Here's how the part is built. I have some questions about the finished solid (model axes, mm). Face numbers are marked on the shaded views. A direction names the side the tool comes from. Round coordinates to 2 decimals unless told otherwise and drop trailing zeros. Write each loop counter-clockwise with the first axis right and the second up, starting at its lowest first coordinate (ties: lowest second). Pieces come first, ordered by that corner, then holes. Notation, with made-up numbers: (-35.75, 44) -> (1.25, 44) arc R5 ccw to (1.25, 52) -> close; hole circle Ø6 at (69, 68). An arc over 180 degrees is marked (long way). Put each result on its own line as item: value. Start each with the question number.
1. Suppose I cut it at D-D (x = 22.5). Please give me the cut outline in (y, z).
2. For pin 1 (1.5 mm diameter, centred on x = -31.5, z = 7.5, fed in from +Y); pin 2 (3.5 mm diameter, centred on y = -1.5, z = 18.5, fed in from -X); pin 3 (2.5 mm diameter, centred on x = 22, y = 1.5, fed in from +Z), each with a flat end and sliding along its axis, tell me the tip position at first contact or that it passes through.
3. Suppose I cut it at C-C (y = -14). Please give me the cut outline in (x, z), then the cut area to 3 significant figures.
4. Suppose I cut it at B-B (z = 9). Count the separate pieces of the cut face and the enclosed holes in it, then the cut area to 3 significant figures.
5. I need wall thicknesses on probe 1 along X at (y, z) = (-18, 11); probe 2 along X at (y, z) = (-14.5, 11.5); probe 3 along X at (y, z) = (-11.75, 1). Which ranges of each line are inside material? Lowest first, please. Write a range as from..to.
6. Suppose I cut it at A-A (y = 0). Please give me the cut outline in (x, z), then the cut area to 3 significant figures.
7. Which directions (+Z, -Z, +X, -X, +Y, -Y) give clear straight access to the entire face, cutting with the end or side of a thin tool? Please do the marked faces 1, 2 and 3.
8. We'd pull the mould along Y, two halves only. Please class the marked faces 4, 5 and 6: +Y half, -Y half, draft (parallel to the pull), parting line (faces both ways), or undercut.
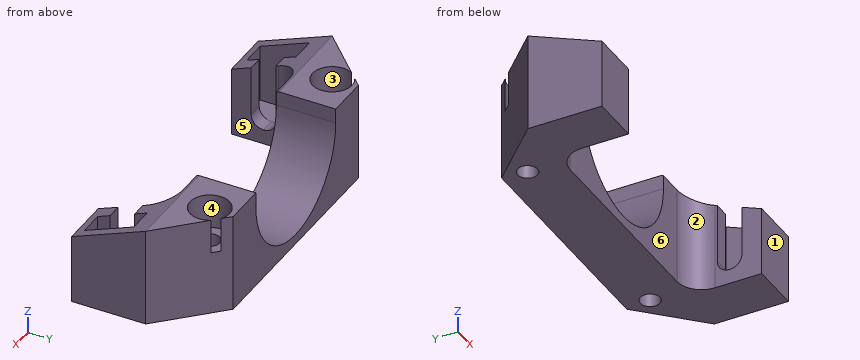
```python
from build123d import *

# Parameters (mm, degrees)
SKETCH1_R               = 2
BOSS_EXTRUDE1_DEPTH     = 20
SKETCH2_W               = 5.5
SKETCH2_H               = 5
SKETCH2_W_2             = 3
SKETCH2_W_3             = 2.5
CUT_EXTRUDE1_DEPTH      = 17
FILLET1_R               = 2.5
FILLET1_OF_MIRROR1_R    = 2.5
CUT_EXTRUDE2_DEPTH      = 43.839817927
CUT_EXTRUDE3_DEPTH      = 46.686431246
CUT_EXTRUDE3_DEPTH_BACK = 46.686431246
SKETCH5_R               = 4
CUT_EXTRUDE4_DEPTH      = 7


with BuildPart() as part:
    # Sketch1 → Boss-Extrude1 (new body)
    with BuildSketch(Plane.XY):
        with BuildLine():
            Line((-23.5, 5), (23.5, 5))
            Line((23.5, 5), (35, -6.5))
            Line((35, -6.5), (35, -21.5))
            Line((35, -21.5), (25, -21.5))
            Line((25, -21.5), (25, -12))
            ThreePointArc((25, -12), (23.535533906, -8.464466094), (20, -7))
            Line((20, -7), (-20, -7))
            ThreePointArc((-20, -7), (-23.535533906, -8.464466094), (-25, -12))
            Line((-25, -12), (-25, -21.5))
            Line((-25, -21.5), (-35, -21.5))
            Line((-35, -21.5), (-35, -6.5))
            Line((-35, -6.5), (-23.5, 5))
        make_face()
        with Locations((-23, 0)):
            Circle(SKETCH1_R, mode=Mode.SUBTRACT)
        with Locations((23, 0)):
            Circle(SKETCH1_R, mode=Mode.SUBTRACT)
    extrude(amount=BOSS_EXTRUDE1_DEPTH)

    # Sketch2 → Cut-Extrude1 (cut)
    with BuildSketch(Plane.XY.offset(20)):
        with Locations((-22.25, -15)):
            Rectangle(SKETCH2_W, SKETCH2_H)
        with Locations((-26.5, -15)):
            Rectangle(SKETCH2_W_2, SKETCH2_H)
        with Locations((-29.25, -15)):
            Rectangle(SKETCH2_W_3, SKETCH2_H)
        Polygon((-30.5, -12.5), (-28, -12.5), (-28, -10), (-33, -10), (-33, -20), (-28, -20), (-28, -17.5), (-30.5, -17.5), align=None)
    cut_extrude1 = extrude(amount=-CUT_EXTRUDE1_DEPTH, mode=Mode.SUBTRACT)

    # Fillet1
    fillet1_edges = [part.edges().sort_by_distance(p)[0] for p in [
        (-26.5, -17.5, 3),
        (-26.5, -12.5, 3),
    ]]
    fillet(fillet1_edges, radius=FILLET1_R - 0.0001)  # a hair under: the kernel refuses the full size

    # Mirror1: Cut-Extrude1 across plane
    add(cut_extrude1.mirror(Plane(origin=(0, 0, 0), x_dir=(0, 0, 1), z_dir=(1, 0, 0))), mode=Mode.SUBTRACT)

    # Fillet1 of Mirror1
    fillet1_of_mirror1_edges = [part.edges().sort_by_distance(p)[0] for p in [
        (26.5, -17.5, 3),
        (26.5, -12.5, 3),
    ]]
    fillet(fillet1_of_mirror1_edges, radius=FILLET1_OF_MIRROR1_R - 0.0001)  # a hair under: the kernel refuses the full size

    # Sketch3 → Cut-Extrude2 (cut, through all)
    with BuildSketch(Plane.XZ.offset(7)):
        with BuildLine():
            Line((-15, 47), (15, 47))
            Line((15, 47), (15, 17))
            ThreePointArc((15, 17), (0, 2), (-15, 17))
            Line((-15, 17), (-15, 47))
        make_face()
    extrude(amount=-CUT_EXTRUDE2_DEPTH, mode=Mode.SUBTRACT)

    # Sketch4 → Cut-Extrude3 (cut, two sides: drawn at the far end of the back side and taken through both)
    with BuildSketch(Plane(origin=(0, 0, 0), x_dir=(0, 0, -1), z_dir=(1, 0, 0)).offset(-CUT_EXTRUDE3_DEPTH_BACK)):
        Polygon((-14, -21.5), (-20, -6.5), (-20, -21.5), align=None)
    extrude(amount=CUT_EXTRUDE3_DEPTH + CUT_EXTRUDE3_DEPTH_BACK, mode=Mode.SUBTRACT)

    # Sketch5 → Cut-Extrude4 (cut)
    with BuildSketch(Plane.XY.offset(20)):
        with Locations((-23, 0)):
            Circle(SKETCH5_R)
        with Locations((23, 0)):
            Circle(SKETCH5_R)
    extrude(amount=-CUT_EXTRUDE4_DEPTH, mode=Mode.SUBTRACT)


solid = part.part
```
Verdict:
1. outline: (-7.67, 0) -> (-1.94, 0) -> (-1.94, 13) -> (-3.97, 13) -> (-3.97, 20) -> (-6.5, 20) -> (-7.67, 19.53) -> close; (1.94, 0) -> (5, 0) -> (5, 20) -> (3.97, 20) -> (3.97, 13) -> (1.94, 13) -> close
2. pin 1: stops at y = -2.25
2. pin 2: stops at x = -31.75
2. pin 3: stops at z = 13
3. outline: (-35, 0) -> (-25, 0) -> (-25, 3.21) -> (-28, 3.21) -> (-28, 3) -> (-33, 3) -> (-33, 17) -> (-35, 17) -> close; (25, 0) -> (35, 0) -> (35, 17) -> (33, 17) -> (33, 3) -> (28, 3) -> (28, 3.21) -> (25, 3.21) -> close
3. area: 117 mm^2
4. separate pieces: 2
4. enclosed holes: 2
4. area: 549 mm^2
5. probe 1: x = -35..-33, -28..-25, 25..28, 33..35
5. probe 2: x = -35..-33, 33..35
5. probe 3: x = -35..-24.99, 24.99..35
6. outline: (-28.5, 0) -> (-25, 0) -> (-25, 13) -> (-27, 13) -> (-27, 20) -> (-28.5, 20) -> close; (-21, 0) -> (21, 0) -> (21, 13) -> (19, 13) -> (19, 20) -> (15, 20) -> (15, 17) arc R15 cw to (-15, 17) -> (-15, 20) -> (-19, 20) -> (-19, 13) -> (-21, 13) -> close; (25, 0) -> (28.5, 0) -> (28.5, 20) -> (27, 20) -> (27, 13) -> (25, 13) -> close
6. area: 481 mm^2
7. face 1: +Z, -Z, +X, -X, -Y
7. face 2: +Z, -Z, -Y
7. face 3: +Z
8. face 4: undercut
8. face 5: draft
8. face 6: -Y half
